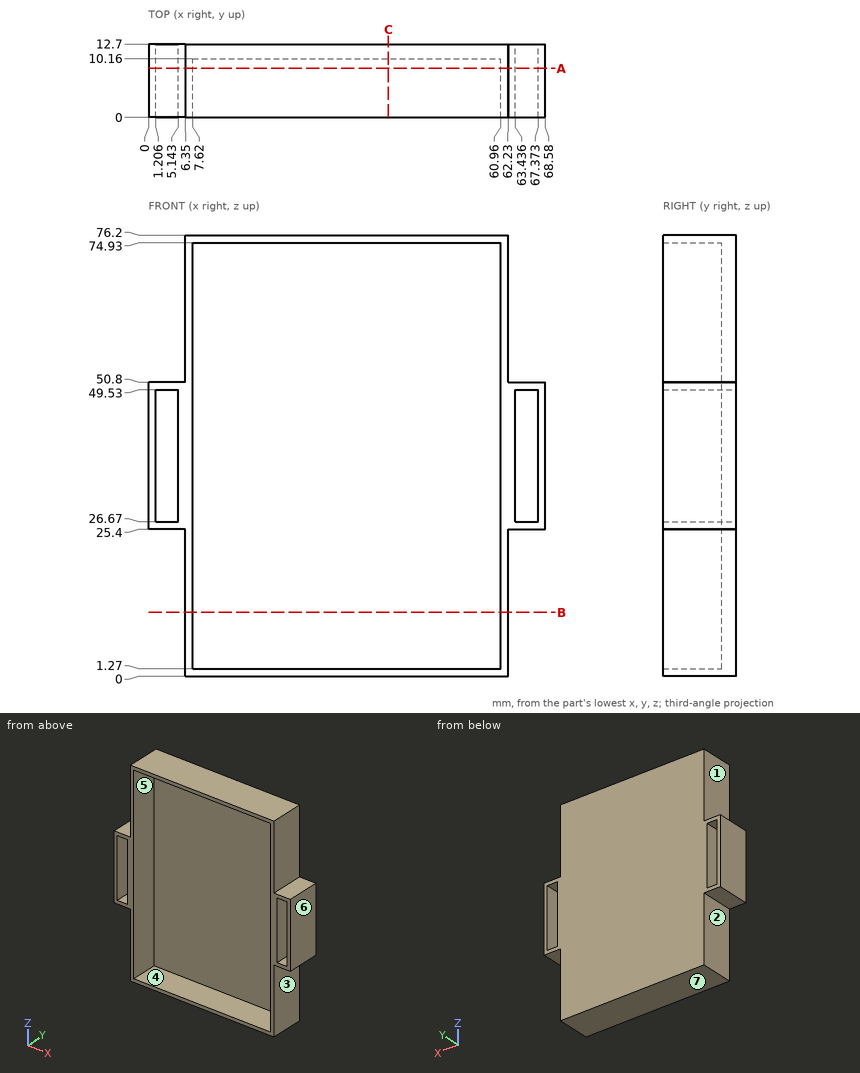
The figure shows three views and two pictorial views of one solid part (mm, origin at its lowest corner). Answer the questions. A direction names the side the tool comes from. Give positions to 0.01 mm unless a question says otherwise; leave off trailing zeros. Loops run counter-clockwise (first coordinate to the right, second up) from the corner with the lowest first, then second, coordinate; pieces in that order, holes last. Notation, with made-up numbers: (32.25, 17) -> (44.25, 17) arc R10 cw to (44.25, 29) -> close; hole circle Ø1 at (89.5, 68.25). An arc over 180 degrees is marked (long way). Use a Markdown table: item, result. Add a question column.
1. Find the intervals of material crossed by probe 1 along X at (y, z) = (0.5, 45); probe 2 along Z at (x, y) = (42, 1.25); probe 3 along X at (y, z) = (8, 6), in increasing order.
2. Section B-B on z = 11 is taken. Determine the outline of the cut face in (x, y), and give its area (3 significant figures).
3. Determine the mould class of the marked faces 5, 6 and 7 for opening direction Z: released by +Z, released by -Z, zero draft, split by the parting line, or undercut.
4. Section C-C on x = 41.5 is taken. Determine the outline of the cut face in (y, z).
5. Flat-ended cylindrical pins translate along their axes: pin 1 Ø1.5 at (x, z) = (43, 15) entering from -Y; pin 2 Ø3 at (x, y) = (64.5, 3) entering from -Z; pin 3 Ø1.2 at (x, y) = (65.5, 4) entering from +Z. Find the tip coordinate at first contact, or state that the pin passes through.
6. For the marked faces 1, 2, 3 and 4, determine the directions among +Z, -Z, +X, -X, +Y, -Y from which every point of the face is accessible in a straight line to the end or side of a thin tool.
7. Section A-A on y = 8.5 is taken. Determine the outline of the cut face in (x, z).
Results below:
| question | item | result |
|---|---|---|
| 1 | probe 1 | x = 0 to 1.21, 5.14 to 7.62, 60.96 to 63.44, 67.37 to 68.58 |
| 1 | probe 2 | z = 0 to 1.27, 74.93 to 76.2 |
| 1 | probe 3 | x = 6.35 to 7.62, 60.96 to 62.23 |
| 2 | outline | (6.35, 0) -> (7.62, 0) -> (7.62, 10.16) -> (60.96, 10.16) -> (60.96, 0) -> (62.23, 0) -> (62.23, 12.7) -> (6.35, 12.7) -> close |
| 2 | area | 168 mm^2 |
| 3 | face 5 | undercut |
| 3 | face 6 | zero draft |
| 3 | face 7 | released by -Z |
| 4 | outline | (0, 0) -> (12.7, 0) -> (12.7, 76.2) -> (0, 76.2) -> (0, 74.93) -> (10.16, 74.93) -> (10.16, 1.27) -> (0, 1.27) -> close |
| 5 | pin 1 | stops at y = 10.16 |
| 5 | pin 2 | stops at z = 25.4 |
| 5 | pin 3 | stops at z = 50.8 |
| 6 | face 1 | +Z, -X, +Y, -Y |
| 6 | face 2 | -Z, -X, +Y, -Y |
| 6 | face 3 | -Z, +X, +Y, -Y |
| 6 | face 4 | -Y |
| 7 | outline | (0, 25.4) -> (6.35, 25.4) -> (6.35, 0) -> (62.23, 0) -> (62.23, 25.4) -> (68.58, 25.4) -> (68.58, 50.8) -> (62.23, 50.8) -> (62.23, 76.2) -> (6.35, 76.2) -> (6.35, 50.8) -> (0, 50.8) -> close; hole (1.21, 26.67) -> (5.14, 26.67) -> (5.14, 49.53) -> (1.21, 49.53) -> close; hole (7.62, 1.27) -> (60.96, 1.27) -> (60.96, 74.93) -> (7.62, 74.93) -> close; hole (63.44, 26.67) -> (67.37, 26.67) -> (67.37, 49.53) -> (63.44, 49.53) -> close |
